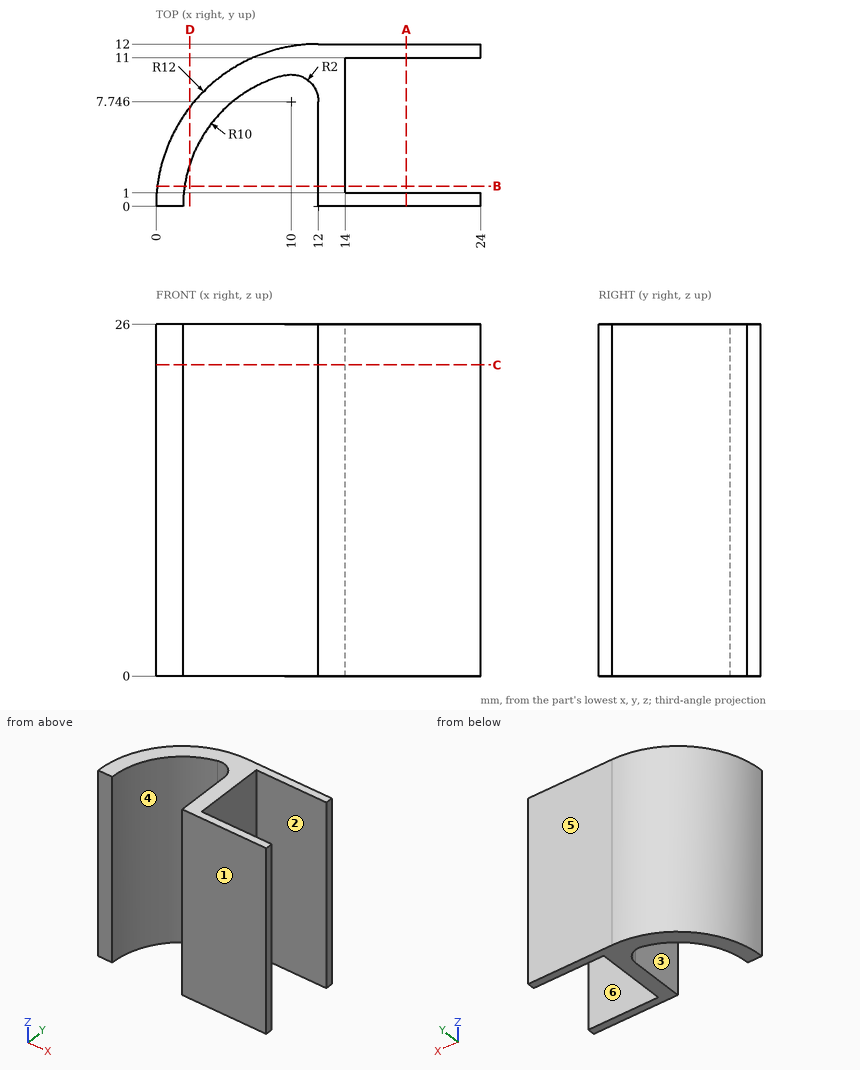
Could you check a few things on this drawing? It's one solid part, dimensions in mm from its lowest x, y, z. A direction names the side the tool comes from. Coordinates: 2 decimals unless noted, no trailing zeros. Loops run counter-clockwise (first coordinate to the right, second up) from the corner with the lowest first, then second, coordinate; pieces in that order, holes last. Notation, with made-up numbers: (39, 18.25) - (47, 18.25) arc R32 ccw to (47, 45.25) - close; hole circle Ø6 at (24.25, 89.5). An arc over 180 degrees is marked (long way). Answer as a JSON object with one key per item and string values. Group by question number.
Item 1: If we section it at A-A (x = 18.5): List the corners of the cut face in (y, z) for me, plus the area to 3 significant figures.
Item 2: On a 3-axis mill with a long thin cutter (end or side, diameter ignored), from which of +Z, -Z, +X, -X, +Y, -Y can I reach the whole of each face in a straight line? I mean the marked faces 4, 5 and 6. Say none if no direction works.
Item 3: If we section it at C-C (z = 23): List the corners of the cut face in (x, y) for me, plus the area to 3 significant figures.
Item 4: If I drill on L1, parallel to Y at x = 16.5, z = 2.75; L2, parallel to X at y = 5.25, z = 12.5; L3, parallel to X at y = 5, z = 2.5, over which ranges is the centre line in solid material (lowest first)? Write a range as from..to.
Item 5: If we section it at B-B (y = 1.5): List the corners of the cut face in (x, z) for me.
Item 6: If we section it at D-D (x = 2.5): List the corners of the cut face in (y, z) for me.
Item 7: If we mould it in two halves opening along Y, with no side actions, what happens to the marked faces 1, 2 and 3? For each: released by +Y, released by -Y, zero draft, split by the parting line, or undercut.
Item 8: For pin 1 (5 mm diameter, centred on y = 5, z = 11.5, fed in from +X); pin 2 (1.5 mm diameter, centred on x = 20, z = 11, fed in from -Y); pin 3 (3 mm diameter, centred on y = 8, z = 5, fed in from -X); pin 4 (6 mm diameter, centred on y = 4.5, z = 11, fed in from -X), each with a flat end and sliding along its axis, tell me the tip position at first contact or that it passes through.
Returned:
{
 "1": {"outline": "(0, 0) - (1, 0) - (1, 26) - (0, 26) - close; (11, 0) - (12, 0) - (12, 26) - (11, 26) - close", "area": "52.0 mm²"},
 "2": {"face 4": "+Z, -Z, -Y", "face 5": "+Z, -Z, +X, -X, +Y", "face 6": "+Z, -Z, +X"},
 "3": {"outline": "(0, 0) - (2, 0) arc R10 cw to (9.5, 9.68) arc R2 cw to (12, 7.75) - (12, 0) - (24, 0) - (24, 1) - (14, 1) - (14, 11) - (24, 11) - (24, 12) - (12, 12) arc R12 ccw to start", "area": "79.8 mm²"},
 "4": {"L1": "y = 0..1, 11..12", "L2": "x = 1.21..3.49, 12..14", "L3": "x = 1.09..3.34, 12..14"},
 "5": {"outline": "(0.09, 0) - (2.11, 0) - (2.11, 26) - (0.09, 26) - close; (12, 0) - (14, 0) - (14, 26) - (12, 26) - close"},
 "6": {"outline": "(3.12, 0) - (7.33, 0) - (7.33, 26) - (3.12, 26) - close"},
 "7": {"face 1": "released by -Y", "face 2": "undercut", "face 3": "zero draft"},
 "8": {"pin 1": "stops at x = 14", "pin 2": "stops at y = 0", "pin 3": "stops at x = 1.91", "pin 4": "stops at x = 0.09"}
}
